CAD build for the part. Positions are in the model's coordinates, mm. A direction names the side the tool comes from. Give positions to 0.01 mm unless a question says otherwise; leave off trailing zeros. Order: outer loops, then holes, each group sorted by start corner. A loop starts at its lowest first (then second) coordinate and runs counter-clockwise, first axis right, second up. Notation, with made-up numbers: (64.5, -34.75) -> (108.5, -34.75) arc R13 ccw to (108.5, -23.75) -> close; hole circle Ø10 at (82.25, -36). An arc over 180 degrees is marked (long way). Answer as CSV lines item,"result".
Autodesk Inventor part; units mm, degrees
ref_plane "YZ Plane" through (0, 0, 0) normal (1, 0, 0) x (0, 1, 0)
ref_plane "XZ Plane" through (0, 0, 0) normal (0, 1, 0) x (-1, 0, 0)
ref_plane "XY Plane" through (0, 0, 0) normal (0, 0, 1) x (1, 0, 0)
sketch "Sketch1" plane through (0, 0, 0) normal (0, 0, 1) x (1, 0, 0)
  line L0 (4.3682, 17.1217) -> (14.3682, 17.1217)
  line L1 (14.3682, 17.1217) -> (14.3682, 2.1217)
  line L2 (14.3682, 2.1217) -> (4.3682, 2.1217)
  line L3 (4.3682, 2.1217) -> (4.3682, 17.1217)
  dimension "d0" = 10
  dimension "d1" = 15
extrude "Extrusion1" add sketch "Sketch1" along normal blind 1.6
sketch "Sketch2" plane through (0, 0, 1.6) normal (0, 0, 1) x (1, 0, 0)
  line L0 (4.3682, 17.1217) -> (14.3682, 17.1217)
  line L1 (4.3682, 2.1217) -> (4.3682, 17.1217)
  circle A0 centre (9.3682, 9.6217) radius 3.45
  dimension "d4" = 6.9
  dimension "d5" = 5
  dimension "d6" = 7.5
extrude "Extrusion2" add sketch "Sketch2" along normal blind 1.4
sketch "Sketch3" plane through (9.3682, 9.6217, 3) normal (0, 0, 1) x (1, 0, 0)
  circle A0 centre (0, 0) radius 3.45
  circle A1 centre (0, 0) radius 2.5
  dimension "d9" = 5
extrude "Extrusion3" cut sketch "Sketch3" against normal through all contours A1
fillet "Fillet1" radius 0.5 4 edges at (14.3682, 17.1217, 0.8) (14.3682, 2.1217, 0.8) (4.3682, 2.1217, 0.8) (4.3682, 17.1217, 0.8)
fillet "Fillet2" radius 0.1 17 edges at (5.9182, 9.6217, 3) (14.3682, 9.6217, 1.6) (14.2217, 2.2681, 1.6) (9.3682, 2.1217, 1.6) (4.5146, 2.2681, 1.6) (4.3682, 9.6217, 1.6) (4.5146, 16.9752, 1.6) (9.3682, 17.1217, 1.6) (14.2217, 16.9752, 1.6) (14.3682, 9.6217, 0) (14.2217, 2.2681, 0) (9.3682, 2.1217, 0) (4.5146, 2.2681, 0) (4.3682, 9.6217, 0) (4.5146, 16.9752, 0) (9.3682, 17.1217, 0) (14.2217, 16.9752, 0)
properties part number "SM-H11" material "Steel, Mild"
1) Band-saw the part on A-A, the plane z = 1. Write the cut outline in (x, y).
Data:
outline,"(4.37, 2.62) arc R0.5 ccw to (4.87, 2.12) -> (13.87, 2.12) arc R0.5 ccw to (14.37, 2.62) -> (14.37, 16.62) arc R0.5 ccw to (13.87, 17.12) -> (4.87, 17.12) arc R0.5 ccw to (4.37, 16.62) -> close; hole circle Ø5 at (9.37, 9.62)"
2) Wall check: line 1 along X through (y, z) = (9.5, 0.7); line 2 along Y through (x, z) = (9.5, 0.6); line 3 along Z through (x, y) = (7.75, 6.5). Give the ranges that are in metal, low to high. Write a range as [from, to].
Data:
line 1,"x = [4.37, 6.87], [11.87, 14.37]"
line 2,"y = [2.12, 7.13], [12.12, 17.12]"
line 3,"z = [0, 1.6]"
3) Pin check, flat tips, straight feed: P1, Ø1.5, axis at x = 11, z = 2.5, coming from the +Y side; P2, Ø6, axis at x = 13, y = 13.5, coming from the -Z side. Stop position of each tip, or through.
Data:
P1,"stops at y = 12.96"
P2,"stops at z = 0"
4) Band-saw the part on C-C, the plane y = 14. Write the cut outline in (x, z), then the cut area to 3 significant figures.
Data:
outline,"(4.37, 0.1) arc R0.1 ccw to (4.47, 0) -> (14.27, 0) arc R0.1 ccw to (14.37, 0.1) -> (14.37, 1.5) arc R0.1 ccw to (14.27, 1.6) -> (4.47, 1.6) arc R0.1 ccw to (4.37, 1.5) -> close"
area,"16.0 mm2"
5) Band-saw the part on D-D, the plane z = 2.2. Write the cut outline in (x, y).
Data:
outline,"circle Ø6.9 at (9.37, 9.62); hole circle Ø5 at (9.37, 9.62)"
6) Band-saw the part on B-B, the plane x = 5.5. Write the cut outline in (y, z), then the cut area to 3 significant figures.
Data:
outline,"(2.12, 0.1) arc R0.1 ccw to (2.22, 0) -> (17.02, 0) arc R0.1 ccw to (17.12, 0.1) -> (17.12, 1.5) arc R0.1 ccw to (17.02, 1.6) -> (2.22, 1.6) arc R0.1 ccw to (2.12, 1.5) -> close"
area,"24.0 mm2"
7) Which spindle directions (+Z, -Z, +X, -X, +Y, -Y) get a long thin tool onto all of the face, cutting with end or side? Do faces 4 (the flat face through (4.368, 10, 1)), 5 (the flat face through (8, 13, 1.6)). Say none if no direction does.
Data:
face 4,"+Z, -Z, -X, +Y, -Y"
face 5,"+Z"
8) Pull direction X, two halves, no side cores. Call faces 1 (the flat face through (14.368, 10, 1)), 2 (the flat face through (11.5, 11.4, 0)), 3 (the cylindrical face through (11.753, 10.373, 1.521)): pulls with the +X half, pulls with the -X half, needs draft (parallel to the pull), parting line crosses it, or undercut.
Data:
face 1,"pulls with the +X half"
face 2,"needs draft"
face 3,"undercut"
